Could you check a few things on this model? Use its own coordinates, in mm. Face numbers are marked on the shaded views. A direction names the side the tool comes from. Give positions to 0.01 mm unless a question says otherwise; leave off trailing zeros. Order: outer loops, then holes, each group sorted by start corner. A loop starts at its lowest first (then second) coordinate and runs counter-clockwise, first axis right, second up. Notation, with made-up numbers: M 54,42 L 104,42 A29 cw 104,74 Z; hole C -3.5,38 d2. An arc over 180 degrees is marked long. Use a Markdown table: item, result. Add a question column.
Item 1: Suppose I cut it at D-D on z = -2.5. Write out the boundary of the cut face in (x, y).
Item 2: If I drill on L1, parallel to Y at x = 1.75, z = -12; L2, parallel to Y at x = 7.5, z = 0; L3, parallel to X at y = -8.5, z = 0.5, over which ranges is the centre line in solid material (lowest first)? Write a range as from..to.
Item 3: Suppose I cut it at C-C on x = 2. Write out the boundary of the cut face in (y, z), plus the area to 3 significant figures.
Item 4: I'm going to push flat-ended pins straight in: pin 1 Ø6 at (x, z) = (18.5, -5) entering from +Y; pin 2 Ø3 at (x, z) = (12.5, -6) entering from +Y; pin 3 Ø4 at (x, z) = (15.5, -8.5) entering from +Y. Where does each tip first touch, or does it pass through?
Item 5: Suppose I cut it at A-A on y = 0. Write out the boundary of the cut face in (x, z), plus the area to 3 significant figures.
Item 6: If we mould it in two halves opening along Y, with no side actions, what happens to the marked faces 1, 2 and 3? For each: released by +Y, released by -Y, zero draft, split by the parting line, or undercut.
Item 7: For the marked faces 4, 5 and 6, which set-ups out of +Z, -Z, +X, -X, +Y, -Y let a thin tool reach every point of the face, with its end or its side?
Item 8: Suppose I cut it at B-B on z = 1.5. Write out the boundary of the cut face in (x, y).
from build123d import *

# Parameters (mm, degrees)
EXTRUDE_3_DEPTH     = 5
SKETCH_3_R          = 2.25
CUT_EXTRUDE_4_DEPTH = 2.5
SKETCH_5_R          = 7.5
EXTRUDE_4_DEPTH     = 18.5
SKETCH_6_R          = 4.5
CUT_EXTRUDE_5_DEPTH = 24.5
SKETCH_7_R          = 3.25
CUT_EXTRUDE_6_DEPTH = 2.5


with BuildPart() as part:
    # 草图1 → 凸台-拉伸3 (new body)
    with BuildSketch(Plane(origin=(0, 0, 0), x_dir=(0, 0, -1), z_dir=(1, 0, 0))):
        with BuildLine():
            Line((-12.072696468, 10.5), (12.072696468, 10.5))
            ThreePointArc((12.072696468, 10.5), (16, 0), (12.072696468, -10.5))
            Line((12.072696468, -10.5), (-12.072696468, -10.5))
            ThreePointArc((-12.072696468, -10.5), (-16, 0), (-12.072696468, 10.5))
        make_face()
    extrude(amount=EXTRUDE_3_DEPTH)

    # 草图3 → 切除-拉伸4 (cut)
    with BuildSketch(Plane(origin=(5, 0, 0), x_dir=(0, 0, -1), z_dir=(1, 0, 0))):
        with Locations((-12, 0)):
            Circle(SKETCH_3_R)
        with Locations((12, 0)):
            Circle(SKETCH_3_R)
    extrude(amount=-CUT_EXTRUDE_4_DEPTH, mode=Mode.SUBTRACT)

    # 草图5 → 凸台-拉伸4 (add)
    with BuildSketch(Plane(origin=(5, 0, 0), x_dir=(0, 0, -1), z_dir=(1, 0, 0))):
        Circle(SKETCH_5_R)
    extrude(amount=EXTRUDE_4_DEPTH)

    # 草图6 → 切除-拉伸5 (cut, through all)
    with BuildSketch(Plane(origin=(23.5, 0, 0), x_dir=(0, 0, -1), z_dir=(1, 0, 0))):
        Circle(SKETCH_6_R)
    extrude(amount=-CUT_EXTRUDE_5_DEPTH, mode=Mode.SUBTRACT)

    # 草图7 → 切除-拉伸6 (cut)
    with BuildSketch(Plane.ZY):
        with Locations((-12, 0)):
            Circle(SKETCH_7_R)
        with Locations((12, 0)):
            Circle(SKETCH_7_R)
    extrude(amount=-CUT_EXTRUDE_6_DEPTH, mode=Mode.SUBTRACT)


solid = part.part
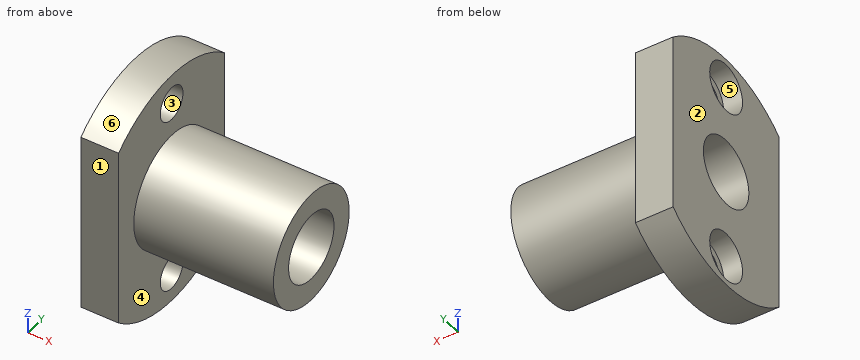
Findings below:
| question | item | result |
|---|---|---|
| 1 | outline | M 0,-10.5 L 5,-10.5 L 5,-7.07 L 23.5,-7.07 L 23.5,-3.74 L 0,-3.74 Z; M 0,3.74 L 23.5,3.74 L 23.5,7.07 L 5,7.07 L 5,10.5 L 0,10.5 Z |
| 2 | L1 | y = -10.5..-3.25, 3.25..10.5 |
| 2 | L2 | y = -7.5..-4.5, 4.5..7.5 |
| 2 | L3 | x = 0..5 |
| 3 | outline | M -10.5,-12.07 A16 ccw 10.5,-12.07 L 10.5,12.07 A16 ccw -10.5,12.07 Z; hole C 0,0 d9; hole C 0,-12 d6.5; hole C 0,12 d6.5 |
| 3 | area | 490 mm^2 |
| 4 | pin 1 | stops at y = 7.23 |
| 4 | pin 2 | stops at y = 6 |
| 4 | pin 3 | stops at y = 3.74 |
| 5 | outline | M 0,-16 L 5,-16 L 5,-14.25 L 2.5,-14.25 L 2.5,-15.25 L 0,-15.25 Z; M 0,-8.75 L 2.5,-8.75 L 2.5,-9.75 L 5,-9.75 L 5,-7.5 L 23.5,-7.5 L 23.5,-4.5 L 0,-4.5 Z; M 0,4.5 L 23.5,4.5 L 23.5,7.5 L 5,7.5 L 5,9.75 L 2.5,9.75 L 2.5,8.75 L 0,8.75 Z; M 0,15.25 L 2.5,15.25 L 2.5,14.25 L 5,14.25 L 5,16 L 0,16 Z |
| 5 | area | 171 mm^2 |
| 6 | face 1 | released by -Y |
| 6 | face 2 | zero draft |
| 6 | face 3 | undercut |
| 7 | face 4 | +X |
| 7 | face 5 | -X |
| 7 | face 6 | +Z, +X, -X |
| 8 | outline | M 0,-10.5 L 5,-10.5 L 5,-7.35 L 23.5,-7.35 L 23.5,-4.24 L 0,-4.24 Z; M 0,4.24 L 23.5,4.24 L 23.5,7.35 L 5,7.35 L 5,10.5 L 0,10.5 Z |
